```python
from build123d import *

# Parameters (mm, degrees)
BOSS_EXTRUDE1_DEPTH = 5.5
SKETCH3_W           = 19.5
SKETCH3_H           = 3
SKETCH3_W_2         = 19.527752912
SKETCH3_H_2         = 8
CUT_EXTRUDE1_DEPTH  = 48.152014803
FILLET1_R           = 1


with BuildPart() as part:
    # Sketch1 → Boss-Extrude1 (new body)
    with BuildSketch(Plane.XY):
        Polygon((39.75, 10), (10.25, 10), (10.25, 8.5), (10.25, 4.646446609), (7.85, 2.246446609), (7.85, 4.975), (6.428553391, 4.975), (4.25, 2.796446609), (4.25, -2.796446609), (6.428553391, -4.975), (7.85, -4.975), (7.85, -2.246446609), (10.25, -4.646446609), (10.25, -8.5), (10.25, -10), (39.75, -10), (39.75, -8.5), (39.75, -4.646446609), (42.15, -2.246446609), (42.15, -4.975), (43.571446609, -4.975), (45.75, -2.796446609), (45.75, 2.796446609), (43.571446609, 4.975), (42.15, 4.975), (42.15, 2.246446609), (39.75, 4.646446609), (39.75, 8.5), align=None)
    extrude(amount=BOSS_EXTRUDE1_DEPTH)

    # Sketch3 → Cut-Extrude1 (cut, through all)
    with BuildSketch(Plane.XY.offset(5.5)):
        with Locations((25, 8.5)):
            Rectangle(SKETCH3_W, SKETCH3_H)
        with Locations((25, -8.5)):
            Rectangle(SKETCH3_W, SKETCH3_H)
        with Locations((25, 0)):
            Rectangle(SKETCH3_W_2, SKETCH3_H_2)
    extrude(amount=-CUT_EXTRUDE1_DEPTH, mode=Mode.SUBTRACT)

    # Fillet1
    fillet1_edges = [part.edges().sort_by_distance(p)[0] for p in [
        (15.25, -10, 2.75),
        (15.25, -7, 2.75),
        (34.75, -7, 2.75),
        (34.75, -10, 2.75),
        (15.236123544, -4, 2.75),
        (15.236123544, 4, 2.75),
        (34.763876456, 4, 2.75),
        (34.763876456, -4, 2.75),
        (10.25, 10, 2.75),
        (39.75, 10, 2.75),
        (39.75, -10, 2.75),
        (10.25, -10, 2.75),
        (15.25, 7, 2.75),
        (15.25, 10, 2.75),
        (34.75, 10, 2.75),
        (34.75, 7, 2.75),
    ]]
    fillet(fillet1_edges, radius=FILLET1_R)


solid = part.part
```
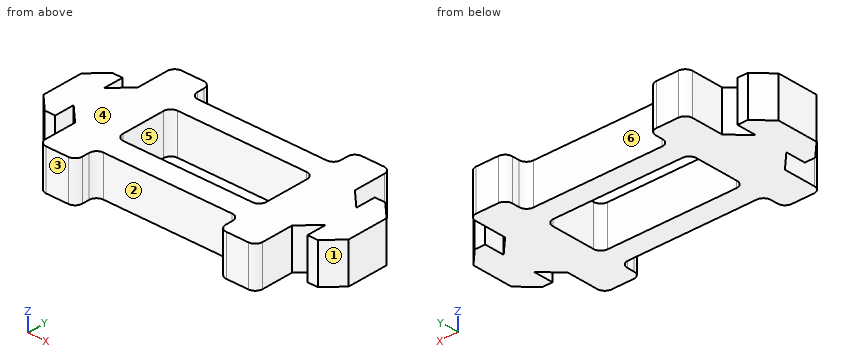
Verification items for the finished model (mm, model axes). Face numbers are marked on the shaded views. A direction names the side the tool comes from. Give positions to 0.01 mm unless a question says otherwise; leave off trailing zeros. Loops run counter-clockwise (first coordinate to the right, second up) from the corner with the lowest first, then second, coordinate; pieces in that order, holes last.
1. Section check B-B, the plane x = 33. Enter the section's corners in (y, z).
2. Section check C-C, the plane y = 5.5. Enter the section's corners in (x, z).
3. Section check A-A, the plane y = 1.75. Enter the section's corners in (x, z).
4. Go/stop test with flat-tipped pins: pin 1 Ø2 at (y, z) = (-4, 1.5) entering from +X; pin 2 Ø3 at (x, z) = (24.5, 4) entering from +Y; pin 3 Ø1.6 at (x, z) = (23.5, 3.5) entering from -Y. Record where each tip stops, or that it passes through.
5. Thickness scan on line 1 (Y direction, x = 21, z = 0.6); line 2 (X direction, y = 1.5, z = 3.6); line 3 (X direction, y = -2.75, z = 0.4). Record the ranges inside material, lowest first.
6. Mould release check, pull along X, two halves, no side actions. Record for the marked faces 1, 2 and 3: released by +X, released by -X, zero draft, split by the parting line, or undercut.
7. Set-up check for the marked faces 4, 5 and 6: record each of +Z, -Z, +X, -X, +Y, -Y from which the full face is reachable in a straight line by a thin tool's end or side.
Geometry says:
1. outline: (-7, 0) - (-4, 0) - (-4, 5.5) - (-7, 5.5) - close; (4, 0) - (7, 0) - (7, 5.5) - (4, 5.5) - close
2. outline: (10.25, 0) - (39.75, 0) - (39.75, 5.5) - (10.25, 5.5) - close
3. outline: (4.25, 0) - (15.24, 0) - (15.24, 5.5) - (4.25, 5.5) - close; (34.76, 0) - (45.75, 0) - (45.75, 5.5) - (34.76, 5.5) - close
4. pin 1: stops at x = 45.55
4. pin 2: stops at y = 7
4. pin 3: stops at y = -7
5. line 1: y = -7 to -4, 4 to 7
5. line 2: x = 4.25 to 15.24, 34.76 to 45.75
5. line 3: x = 4.25 to 7.85, 8.35 to 15.24, 34.76 to 41.65, 42.15 to 45.75
6. face 1: released by +X
6. face 2: undercut
6. face 3: zero draft
7. face 4: +Z, +X, -X, +Y, -Y
7. face 5: +Z, -Z
7. face 6: +Z, -Z, +Y
